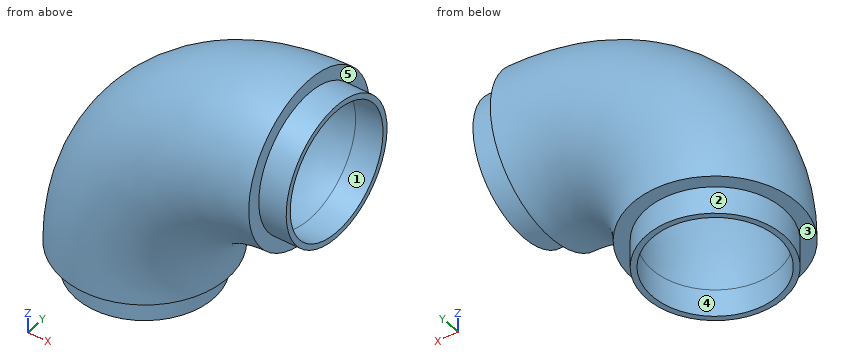
Autodesk Inventor part; units mm, degrees
ref_plane "YZ Plane" through (0, 0, 0) normal (1, 0, 0) x (0, 1, 0)
ref_plane "XZ Plane" through (0, 0, 0) normal (0, 1, 0) x (-1, 0, 0)
ref_plane "XY Plane" through (0, 0, 0) normal (0, 0, 1) x (1, 0, 0)
sketch "Esquisse15" plane through (0, 0, 0) normal (1, 0, 0) x (0, 1, 0)
  circle A0 centre (0, 60) radius 30
  circle A1 centre (0, 60) radius 23
  line L0 (-42, 0) -> (42, 0) construction
  line L1 (0, 108) -> (0, -18) construction
  point P0 (0, 0)
  dimension "d43" = 60
  dimension "d44" = 46
  dimension "d45" = 60
sketch "Esquisse9" plane through (0, 0, 0) normal (0, 1, 0) x (-1, 0, 0)
  arc A0 (60, 0) -> (0, 60) centre (0, 0) ccw
  dimension "d41" = 90
  dimension "d42" = 60
sweep "Balayage3" add profiles "Esquisse15" path "Esquisse9"
sketch "Esquisse16" plane through (-60, 0, 0) normal (0, 0, -1) x (-1, 0, 0)
  circle A0 centre (0, 0) radius 23 construction
  circle A1 centre (0, 0) radius 30 construction
  circle A2 centre (0, 0) radius 23
  circle A3 centre (0, 0) radius 25
  point P0 (-60, 0)
  dimension "d48" = 50
extrude "Extrusion6" add sketch "Esquisse16" along normal blind 10
sketch "Esquisse17" plane through (0, 0, 60) normal (1, 0, 0) x (0, 0, -1)
  circle A0 centre (0, 0) radius 23 construction
  circle A1 centre (0, 0) radius 30 construction
  circle A2 centre (0, 0) radius 23
  circle A3 centre (0, 0) radius 25
  point P0 (60, 0)
  dimension "d51" = 50
extrude "Extrusion7" add sketch "Esquisse17" along normal blind 10
properties part number "P010_CanonCoude"
For this review, take the finished solid that the model builds, in its own axes (mm). Face numbers are marked on the shaded views. A direction names the side the tool comes from. Round coordinates to 2 decimals unless told otherwise and drop trailing zeros. Write each loop counter-clockwise with the first axis right and the second up, starting at its lowest first coordinate (ties: lowest second). Pieces come first, ordered by that corner, then holes. Notation, with made-up numbers: (-13.5, 83) - (15.5, 83) arc R23 ccw to (15.5, 109) - close; hole circle Ø1 at (31.5, 65.5). An arc over 180 degrees is marked (long way). Write item = value, one per line. Start each with the question number.
1. Draft analysis for pull direction X (two halves, no side actions). For the marked faces 3, 4 and 5, state which applies: released by +X, released by -X, zero draft, split by the parting line, or undercut.
2. For the marked faces 1 and 2, list the 3-axis set-ups (+Z, -Z, +X, -X, +Y, -Y) from which the entire face can be reached by the end or side of a thin tool; tool diameter is ignored.
3. For pin 1 Ø4 at (y, z) = (-17.5, 72) entering from -X; pin 2 Ø3 at (y, z) = (-23.5, 14) entering from -X; pin 3 Ø12 at (x, z) = (-39, 76.5) entering from +Y, all flat-tipped, find the tip position at first contact; note any pin that passes through.
4. Consider section B-B on y = -11. State the section outline as (x, z) points, plus the area to 3 significant figures.
5. Consider section A-A on y = 0. State the section outline as (x, z) points.
6. Wall thickness on L1, parallel to Y at x = 2.75, z = 60; L2, parallel to Z at x = -7.5, y = -7; L3, parallel to Z at x = -30.5, y = -14: over which ranges is each line inside the solid? List them lowest first.
Evaluation:
q1.face_3 = zero draft
q1.face_4 = undercut
q1.face_5 = released by +X
q2.face_1 = +X
q2.face_2 = -Z
q3.pin_1 = -47.96
q3.pin_2 = -79.19
q3.pin_3 = 22.48
q4.outline = (-87.91, 0) - (-82.45, 0) - (-82.45, -10) - (-80.2, -10) - (-80.2, 0) arc R80.2 cw to (0, 80.2) - (10, 80.2) - (10, 82.45) - (0, 82.45) - (0, 87.91) arc R87.91 ccw to start; (-39.8, -10) - (-37.55, -10) - (-37.55, 0) - (-32.09, 0) arc R32.09 cw to (0, 32.09) - (0, 37.55) - (10, 37.55) - (10, 39.8) - (0, 39.8) arc R39.8 ccw to (-39.8, 0) - close
q4.area = 1,540 mm2
q5.outline = (-90, 0) - (-85, 0) - (-85, -10) - (-83, -10) - (-83, 0) arc R83 cw to (0, 83) - (10, 83) - (10, 85) - (0, 85) - (0, 90) arc R90 ccw to start; (-37, -10) - (-35, -10) - (-35, 0) - (-30, 0) arc R30 cw to (0, 30) - (0, 35) - (10, 35) - (10, 37) - (0, 37) arc R37 ccw to (-37, 0) - close
q6.L1 = -25 to -23, 23 to 25
q6.L2 = 29.9 to 37.35, 81.56 to 88.86
q6.L3 = 13.78 to 28.51, 72.06 to 80.98
